from build123d import *

# Parameters (mm, degrees)
SKETCH2_R           = 5
BOSS_EXTRUDE1_DEPTH = 10


with BuildPart() as part:
    # Sketch2 → Boss-Extrude1 (new body)
    with BuildSketch(Plane.XY):
        with BuildLine():
            ThreePointArc((49, 9.949874371), (43.301270189, 25), (33.11684397, 37.4603076))
            ThreePointArc((33.11684397, 37.4603076), (30, 51.961524227), (15.88315603, 47.410181971))
            ThreePointArc((15.88315603, 47.410181971), (0, 50), (-15.88315603, 47.410181971))
            ThreePointArc((-15.88315603, 47.410181971), (-30, 51.961524227), (-33.11684397, 37.4603076))
            ThreePointArc((-33.11684397, 37.4603076), (-43.301270189, 25), (-49, 9.949874371))
            ThreePointArc((-49, 9.949874371), (-60, 0), (-49, -9.949874371))
            ThreePointArc((-49, -9.949874371), (-43.301270189, -25), (-33.11684397, -37.4603076))
            ThreePointArc((-33.11684397, -37.4603076), (-30, -51.961524227), (-15.88315603, -47.410181971))
            ThreePointArc((-15.88315603, -47.410181971), (0, -50), (15.88315603, -47.410181971))
            ThreePointArc((15.88315603, -47.410181971), (30, -51.961524227), (33.11684397, -37.4603076))
            ThreePointArc((33.11684397, -37.4603076), (43.301270189, -25), (49, -9.949874371))
            ThreePointArc((49, -9.949874371), (60, 0), (49, 9.949874371))
        make_face()
        with Locations((50, 0)):
            Circle(SKETCH2_R, mode=Mode.SUBTRACT)
        with Locations((25, -43.301270189)):
            Circle(SKETCH2_R, mode=Mode.SUBTRACT)
        with Locations((-25, -43.301270189)):
            Circle(SKETCH2_R, mode=Mode.SUBTRACT)
        with Locations((-50, 0)):
            Circle(SKETCH2_R, mode=Mode.SUBTRACT)
        with Locations((-25, 43.301270189)):
            Circle(SKETCH2_R, mode=Mode.SUBTRACT)
        with Locations((25, 43.301270189)):
            Circle(SKETCH2_R, mode=Mode.SUBTRACT)
    extrude(amount=BOSS_EXTRUDE1_DEPTH)


solid = part.part
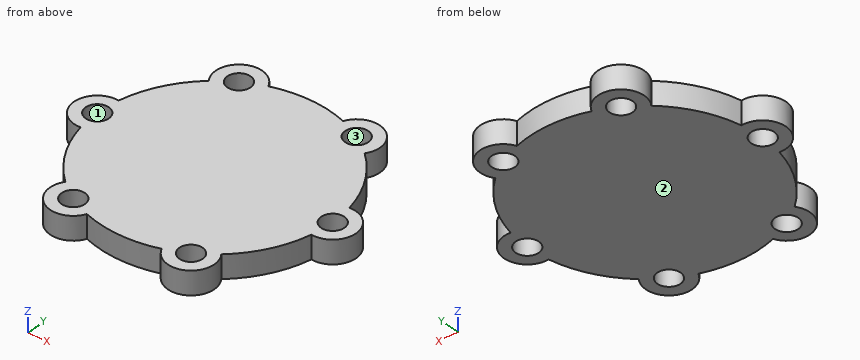
CAD build for the part. Positions are in the model's coordinates, mm. Face numbers are marked on the shaded views. Round coordinates to 2 decimals unless told otherwise and drop trailing zeros. Write each loop counter-clockwise with the first axis right and the second up, starting at its lowest first coordinate (ties: lowest second). Pieces come first, ordered by that corner, then holes. Notation, with made-up numbers: M 77.5,76 L 117.5,76 A33 cw 117.5,106 Z; hole C 31,17 d9. An arc over 180 degrees is marked long. Use a Markdown table: item, result. Add a question column.
1. Drill centre lines: probe 1 along Y at (x, z) = (-25, 6.75); probe 2 along Y at (x, z) = (-50, 6.25); probe 3 along X at (y, z) = (1, 9). Where is each one in solid material? Low to high.
2. Slice it at B-B on y = 0. Give the cut face in (x, z).
3. Slice it at A-A on x = 25. Give the cut face in (y, z).
4. Pull direction X, two halves, no side cores. Call the marked faces 1, 2 and 3: released by +X, released by -X, zero draft, split by the parting line, or undercut.
5. Slice it at D-D on x = -41. Give the cut face in (y, z), then the cut area to 3 significant figures.
6. Flat gauge pins, fed straight in: P1, Ø1, axis at y = 35.5, z = 3, coming from the -X side; P2, Ø9, axis at x = -50, y = 0, coming from the +Z side; P3, Ø4, axis at x = -21, z = 4, coming from the +Y side; P4, Ø2, axis at y = 31, z = 4.5, coming from the +X side. Where does each tip first touch, or does it go through?
7. Slice it at C-C on z = 3. Give the cut face in (x, y), then the cut area to 3 significant figures.
Reply:
| question | item | result |
|---|---|---|
| 1 | probe 1 | y = -53.3 to -48.3, -38.3 to 38.3, 48.3 to 53.3 |
| 1 | probe 2 | y = -10 to -5, 5 to 10 |
| 1 | probe 3 | x = -59.95 to -54.9, -45.1 to 45.1, 54.9 to 59.95 |
| 2 | outline | M -60,0 L -55,0 L -55,10 L -60,10 Z; M -45,0 L 45,0 L 45,10 L -45,10 Z; M 55,0 L 60,0 L 60,10 L 55,10 Z |
| 3 | outline | M -53.3,0 L -48.3,0 L -48.3,10 L -53.3,10 Z; M -38.3,0 L 38.3,0 L 38.3,10 L -38.3,10 Z; M 48.3,0 L 53.3,0 L 53.3,10 L 48.3,10 Z |
| 4 | face 1 | undercut |
| 4 | face 2 | zero draft |
| 4 | face 3 | undercut |
| 5 | outline | M -28.62,0 L 28.62,0 L 28.62,10 L -28.62,10 Z |
| 5 | area | 572 mm^2 |
| 6 | P1 | stops at x = -35.71 |
| 6 | P2 | passes through |
| 6 | P3 | stops at y = 53.1 |
| 6 | P4 | stops at x = 40 |
| 7 | outline | M -49,-9.95 A50 ccw -33.12,-37.46 A10 ccw long -15.88,-47.41 A50 ccw 15.88,-47.41 A10 ccw long 33.12,-37.46 A50 ccw 49,-9.95 A10 ccw long 49,9.95 A50 ccw 33.12,37.46 A10 ccw long 15.88,47.41 A50 ccw -15.88,47.41 A10 ccw long -33.12,37.46 A50 ccw -49,9.95 A10 ccw long Z; hole C -50,0 d10; hole C -25,-43.3 d10; hole C -25,43.3 d10; hole C 25,-43.3 d10; hole C 25,43.3 d10; hole C 50,0 d10 |
| 7 | area | 8,370 mm^2 |
